from build123d import *

# Parameters (mm, degrees)
ESBO_O1_R                = 3.5
ESBO_O1_R_2              = 3
ESBO_O1_R_3              = 1.6
RESSALTO_EXTRUS_O1_DEPTH = 3
ESBO_O2_R                = 1.6
RESSALTO_EXTRUS_O2_DEPTH = 3
FILETE2_R                = 10
CORTE_EXTRUS_O1_DEPTH    = 203.904924863


with BuildPart() as part:
    # Esboço1 → Ressalto-extrusão1 (new body)
    with BuildSketch(Plane(origin=(0, 0, 0), x_dir=(1, 0, 0), z_dir=(0, 1, 0))):
        with BuildLine():
            Line((188.965018959, -38.648697641), (188.965018959, 28))
            ThreePointArc((188.965018959, 28), (185.450300333, 36.485281374), (176.965018959, 40))
            Line((176.965018959, 40), (-176.090826953, 40))
            ThreePointArc((-176.090826953, 40), (-184.576108327, 36.485281374), (-188.090826953, 28))
            Line((-188.090826953, 28), (-188.090826953, -38.648697641))
            ThreePointArc((-188.090826953, -38.648697641), (-184.576108327, -47.133979015), (-176.090826953, -50.648697641))
            Line((-176.090826953, -50.648697641), (176.965018959, -50.648697641))
            ThreePointArc((176.965018959, -50.648697641), (185.450300333, -47.133979015), (188.965018959, -38.648697641))
        make_face()
        with Locations(Location((-62.734509176, 0, 0), (0, 0, 90))):
            Circle(ESBO_O1_R, mode=Mode.SUBTRACT)
        with Locations(Location((176.748138959, -38.431817641, 0), (0, 0, 90))):
            Circle(ESBO_O1_R_2, mode=Mode.SUBTRACT)
        with Locations(Location((0.437096003, -38.431817641, 0), (0, 0, 90))):
            Circle(ESBO_O1_R_2, mode=Mode.SUBTRACT)
        with Locations(Location((79.965018959, 10, 0), (0, 0, 90))):
            Circle(ESBO_O1_R_2, mode=Mode.SUBTRACT)
        with Locations(Location((-140.090826953, 10, 0), (0, 0, 90))):
            Circle(ESBO_O1_R, mode=Mode.SUBTRACT)
        with Locations(Location((-148.090826953, 0, 0), (0, 0, 270))):
            Circle(ESBO_O1_R_3, mode=Mode.SUBTRACT)
        with Locations(Location((-132.090826953, 0, 0), (0, 0, 270))):
            Circle(ESBO_O1_R_3, mode=Mode.SUBTRACT)
        with Locations(Location((-132.090826953, 20, 0), (0, 0, 270))):
            Circle(ESBO_O1_R_3, mode=Mode.SUBTRACT)
        with Locations(Location((-148.090826953, 20, 0), (0, 0, 270))):
            Circle(ESBO_O1_R_3, mode=Mode.SUBTRACT)
        with Locations(Location((-70.734509176, -10, 0), (0, 0, 270))):
            Circle(ESBO_O1_R_3, mode=Mode.SUBTRACT)
        with Locations(Location((-70.734509176, 10, 0), (0, 0, 270))):
            Circle(ESBO_O1_R_3, mode=Mode.SUBTRACT)
        with Locations(Location((-54.734509176, 10, 0), (0, 0, 270))):
            Circle(ESBO_O1_R_3, mode=Mode.SUBTRACT)
        with Locations(Location((-54.734509176, -10, 0), (0, 0, 270))):
            Circle(ESBO_O1_R_3, mode=Mode.SUBTRACT)
        with Locations(Location((-83.930342624, 32.5, 0), (0, 0, 90))):
            Circle(ESBO_O1_R_2, mode=Mode.SUBTRACT)
        with Locations(Location((-175.873946953, -38.431817641, 0), (0, 0, 90))):
            Circle(ESBO_O1_R_2, mode=Mode.SUBTRACT)
        with Locations(Location((140.965018959, 10, 0), (0, 0, 90))):
            Circle(ESBO_O1_R, mode=Mode.SUBTRACT)
        with Locations(Location((148.965018959, 0, 0), (0, 0, 90))):
            Circle(ESBO_O1_R_3, mode=Mode.SUBTRACT)
        with Locations(Location((148.965018959, 20, 0), (0, 0, 90))):
            Circle(ESBO_O1_R_3, mode=Mode.SUBTRACT)
        with Locations(Location((132.965018959, 0, 0), (0, 0, 90))):
            Circle(ESBO_O1_R_3, mode=Mode.SUBTRACT)
        with Locations(Location((132.965018959, 20, 0), (0, 0, 90))):
            Circle(ESBO_O1_R_3, mode=Mode.SUBTRACT)
        with Locations(Location((-181.090826953, -27.648697641, 0), (0, 0, 270))):
            Circle(ESBO_O1_R_3, mode=Mode.SUBTRACT)
    extrude(amount=-RESSALTO_EXTRUS_O1_DEPTH)

    # Esboço2 → Ressalto-extrusão2 (add)
    with BuildSketch(Plane.XZ.offset(3)):
        with BuildLine():
            Line((125.022883335, 50.648697641), (176.965018959, 50.648697641))
            ThreePointArc((176.965018959, 50.648697641), (185.450300333, 47.133979015), (188.965018959, 38.648697641))
            Line((188.965018959, 38.648697641), (188.965018959, 68.848697641))
            ThreePointArc((188.965018959, 68.848697641), (183.965018959, 73.848697641), (178.965018959, 68.848697641))
            Line((178.965018959, 68.848697641), (143.222883335, 68.848697641))
            Line((143.222883335, 68.848697641), (125.022883335, 50.648697641))
        make_face()
        with BuildLine():
            Line((147.365018959, 58.848697641), (181.365018959, 58.848697641))
            ThreePointArc((181.365018959, 58.848697641), (183.965018959, 56.248697641), (181.365018959, 53.648697641))
            Line((181.365018959, 53.648697641), (147.365018959, 53.648697641))
            ThreePointArc((147.365018959, 53.648697641), (144.765018959, 56.248697641), (147.365018959, 58.848697641))
        make_face(mode=Mode.SUBTRACT)
        with Locations(Location((183.965018959, 68.848697641, 0), (0, 0, 270))):
            Circle(ESBO_O2_R, mode=Mode.SUBTRACT)
    extrude(amount=-RESSALTO_EXTRUS_O2_DEPTH)

    # Filete2
    filete2_edges = [part.edges().sort_by_distance(p)[0] for p in [
        (125.022883335, -1.5, 50.648697641),
        (143.222883335, -1.5, 68.848697641),
        (178.965018959, -1.5, 68.848697641),
    ]]
    fillet(filete2_edges, radius=FILETE2_R)

    # Esboço3 → Corte-extrusão1 (cut, through all)
    with BuildSketch(Plane(origin=(0, 0, 0), x_dir=(1, 0, 0), z_dir=(0, 1, 0))):
        with BuildLine():
            Line((-4.234509176, 2.700055346), (-4.234509176, -20.299944654))
            ThreePointArc((-4.234509176, -20.299944654), (-7.734509176, -23.799944654), (-11.234509176, -20.299944654))
            Line((-11.234509176, -20.299944654), (-11.234509176, 2.700055346))
            ThreePointArc((-11.234509176, 2.700055346), (-7.734509176, 6.200055346), (-4.234509176, 2.700055346))
        make_face()
        with BuildLine():
            Line((3.865490824, 10.700055346), (3.865490824, -12.299944654))
            ThreePointArc((3.865490824, -12.299944654), (2.265490824, -13.899944654), (0.665490824, -12.299944654))
            Line((0.665490824, -12.299944654), (0.665490824, 10.700055346))
            ThreePointArc((0.665490824, 10.700055346), (2.265490824, 12.300055346), (3.865490824, 10.700055346))
        make_face()
        with BuildLine():
            Line((3.865490824, -5.299944654), (3.865490824, -28.299944654))
            ThreePointArc((3.865490824, -28.299944654), (2.265490824, -29.899944654), (0.665490824, -28.299944654))
            Line((0.665490824, -28.299944654), (0.665490824, -5.299944654))
            ThreePointArc((0.665490824, -5.299944654), (2.265490824, -3.699944654), (3.865490824, -5.299944654))
        make_face()
        with BuildLine():
            Line((-19.334509176, 10.700055346), (-19.334509176, -12.299944654))
            ThreePointArc((-19.334509176, -12.299944654), (-17.734509176, -13.899944654), (-16.134509176, -12.299944654))
            Line((-16.134509176, -12.299944654), (-16.134509176, 10.700055346))
            ThreePointArc((-16.134509176, 10.700055346), (-17.734509176, 12.300055346), (-19.334509176, 10.700055346))
        make_face()
        with BuildLine():
            Line((-19.334509176, -5.299944654), (-19.334509176, -28.299944654))
            ThreePointArc((-19.334509176, -28.299944654), (-17.734509176, -29.899944654), (-16.134509176, -28.299944654))
            Line((-16.134509176, -28.299944654), (-16.134509176, -5.299944654))
            ThreePointArc((-16.134509176, -5.299944654), (-17.734509176, -3.699944654), (-19.334509176, -5.299944654))
        make_face()
    extrude(amount=-CORTE_EXTRUS_O1_DEPTH, mode=Mode.SUBTRACT)


solid = part.part
The listing builds one solid part. Answer for the finished solid, in the listing's coordinates (mm). Give positions to 0.01 mm unless a question says otherwise; leave off trailing zeros. Use a Markdown table: item, result.
(1) Section A-A, the plane y = -2.3 is taken. Give the number of separate pieces and of enclosed holes in the cut face, then the cut area to 3 significant figures.
Return value:
| item | result |
|---|---|
| separate pieces | 1 |
| enclosed holes | 26 |
| area | 34,100 mm2 |
(2) Flat-ended cylindrical pins translate along their axes: P1, Ø5, axis at x = 148.97, z = -20, coming from the -Y side; P2, Ø1.5, axis at x = 168.5, y = -1, coming from the +Z side. Find the tip coordinate at first contact, or state that the pin passes through.
Return value:
| item | result |
|---|---|
| P1 | y = -3 |
| P2 | z = 68.85 |
(3) Find the intervals of material crossed by probe 1 along Z at (x, y) = (159.5, -0.05); probe 2 along X at (y, z) = (-0.35, 24); probe 3 along X at (y, z) = (-1.6, 40.5), in increasing order. Write a range as from..to.
Return value:
| item | result |
|---|---|
| probe 1 | -40..53.65, 58.85..68.85 |
| probe 2 | -188.09..-19.33, -16.13..0.67, 3.87..188.97 |
| probe 3 | -187.95..-178.05, -173.7..-1.74, 2.61..174.57, 178.92..188.97 |
(4) Determine the mould class of faces 1 (the cylindrical face through (0.31, -1.48, 41.43)), 2 (the flat face through (-2, -3, 5)), 3 (the flat face through (134.209, -1.521, 59.835)) for opening direction X: released by +X, released by -X, zero draft, split by the parting line, or undercut.
Return value:
| item | result |
|---|---|
| face 1 | undercut |
| face 2 | zero draft |
| face 3 | released by -X |
